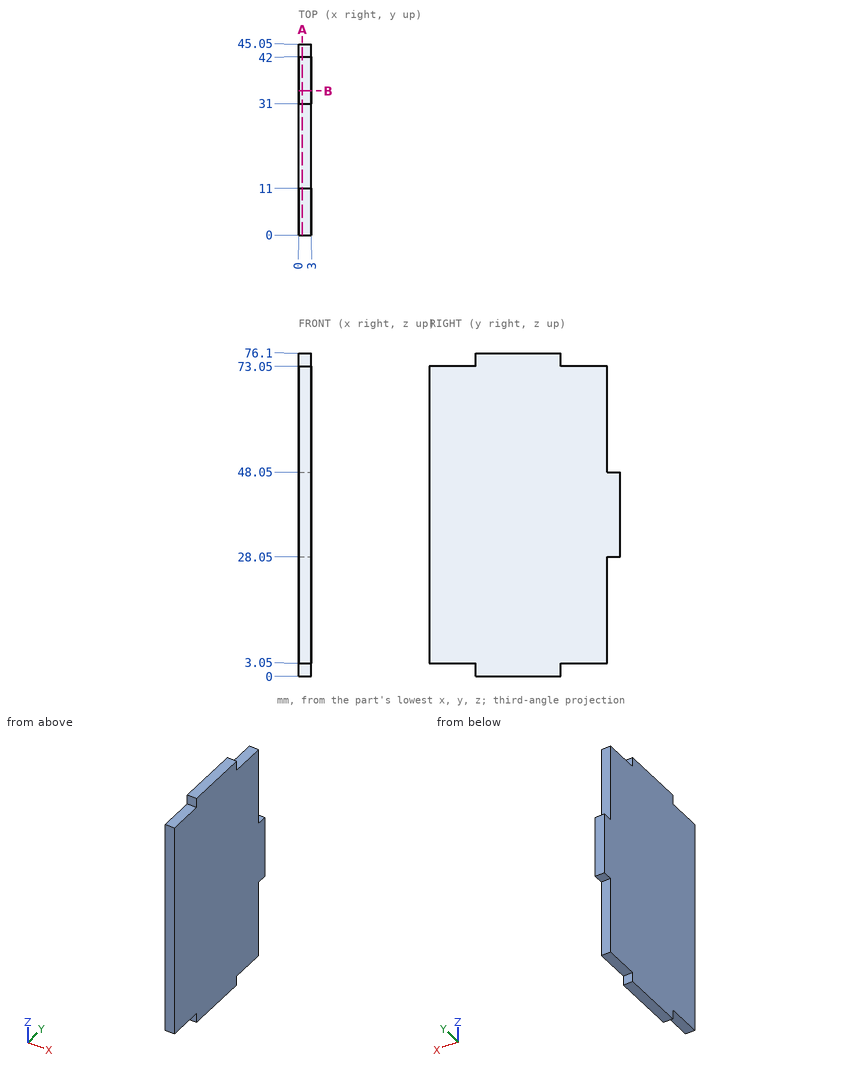
For this review, use the dimensioned drawing (mm, ordinates from the lowest corner) and the shaded views. Round coordinates to 2 decimals unless told otherwise and drop trailing zeros. Write each loop counter-clockwise with the first axis right and the second up, starting at its lowest first coordinate (ties: lowest second). Pieces come first, ordered by that corner, then holes. Notation, with made-up numbers: (2.25, -19.5) -> (7.25, -19.5) arc R11 ccw to (7.25, -5.5) -> close; hole circle Ø10 at (88.25, 43.25). An arc over 180 degrees is marked (long way). Use one line per item in the form item = value.
Q1. Consider section B-B (y = 34). State the section outline as (x, z) points.
Resolved:
outline = (0, 3.05) -> (3, 3.05) -> (3, 73.05) -> (0, 73.05) -> close
Q2. Consider section A-A (x = 0.9). State the section outline as (y, z) points, then the cut area to 3 significant figures.
Resolved:
outline = (0, 3.05) -> (11, 3.05) -> (11, 0) -> (31, 0) -> (31, 3.05) -> (42, 3.05) -> (42, 28.05) -> (45.05, 28.05) -> (45.05, 48.05) -> (42, 48.05) -> (42, 73.05) -> (31, 73.05) -> (31, 76.1) -> (11, 76.1) -> (11, 73.05) -> (0, 73.05) -> close
area = 3,120 mm²
Q3. To check wall thickness, follow probe 1 along Y at (x, z) = (0.9, 22); probe 2 along Z at (x, y) = (2.8, 43.5); probe 3 along Z at (x, y) = (1.25, 31.5). State the ranges of each line that lie inside material, in increasing order. Write a range as from..to.
Resolved:
probe_1 = 0..42
probe_2 = 28.05..48.05
probe_3 = 3.05..73.05
Q4. Clearance check with flat-ended pins moving along their axes: pin 1 Ø1.5 at (x, y) = (2, 9.5) entering from +Z; pin 2 Ø0.9 at (x, y) = (1, 43.5) entering from +Z; pin 3 Ø1.5 at (x, z) = (1.5, 1) entering from +Y. State where each tip first meets the part, or that it passes through.
Resolved:
pin_1 = 73.05
pin_2 = 48.05
pin_3 = 31
